Verification items for the finished model (mm, model axes). A direction names the side the tool comes from. Round coordinates to 2 decimals unless told otherwise and drop trailing zeros. Write each loop counter-clockwise with the first axis right and the second up, starting at its lowest first coordinate (ties: lowest second). Pieces come first, ordered by that corner, then holes. Notation, with made-up numbers: M -36,53.5 L -30,53.5 A33 ccw -30,83.5 Z; hole C 72.5,-24 d10. An arc over 180 degrees is marked long. One line per question, with ' | ' between items.
from build123d import *

# Parameters (mm, degrees)
F0_W     = 48.26
F0_H     = 38.1
F1_DEPTH = 15.24
F3_T     = -0.254
F4_D     = 6.858
F6_D     = 5.08
F7_W     = 8.128
F7_H     = 3.048
F8_DEPTH = 25.4


with BuildPart() as f1:
    # F0 (on Front) → F1 (new body)
    with BuildSketch(Plane.XZ):
        Rectangle(F0_W, F0_H)
    extrude(amount=F1_DEPTH)

    # F3
    f3_openings = [f1.faces().sort_by_distance(p)[0] for p in [
        (0, 0, 0),
    ]]
    offset(amount=F3_T, openings=f3_openings)

    # F4 (through all)
    with Locations(Plane.XZ.offset(15.24)):
        with Locations((-16.383, 0)):
            Hole(F4_D / 2)

    # F6 (through all)
    with Locations(Plane.XZ.offset(15.24)):
        with Locations((0, 0)):
            Hole(F6_D / 2)

    # F7 (on face) → F8 (cut)
    with BuildSketch(Plane.XY.offset(19.05)):
        with Locations((16.256, -11.051697)):
            Rectangle(F7_W, F7_H)
    extrude(amount=-F8_DEPTH, mode=Mode.SUBTRACT)


solid = f1.part
1. Section check C-C, the plane y = -3.5. Record the cut outline in (x, z).
Results:
outline: M -24.13,-19.05 L 24.13,-19.05 L 24.13,19.05 L -24.13,19.05 Z; hole M -23.88,-18.8 L 23.88,-18.8 L 23.88,18.8 L -23.88,18.8 Z
2. Section check D-D, the plane x = -9.5. Record the cut outline in (y, z), then the cut area to 3 significant figures.
Results:
outline: M -15.24,-19.05 L 0,-19.05 L 0,-18.8 L -14.99,-18.8 L -14.99,18.8 L 0,18.8 L 0,19.05 L -15.24,19.05 Z | area: 17.3 mm2
3. Section check B-B, the plane x = 0. Record the cut outline in (y, z).
Results:
outline: M -15.24,-19.05 L 0,-19.05 L 0,-18.8 L -14.99,-18.8 L -14.99,-2.54 L -15.24,-2.54 Z; M -15.24,2.54 L -14.99,2.54 L -14.99,18.8 L 0,18.8 L 0,19.05 L -15.24,19.05 Z
4. Section check A-A, the plane z = 0. Record the cut outline in (x, y), then the cut area to 3 significant figures.
Results:
outline: M -24.13,-15.24 L -19.81,-15.24 L -19.81,-14.99 L -23.88,-14.99 L -23.88,0 L -24.13,0 Z; M -12.95,-15.24 L -2.54,-15.24 L -2.54,-14.99 L -12.95,-14.99 Z; M 2.54,-15.24 L 24.13,-15.24 L 24.13,0 L 23.88,0 L 23.88,-14.99 L 2.54,-14.99 Z | area: 16.8 mm2
5. Mould release check, pull along Z, two halves, no side actions. Record for faces 3 (the face through (-24.13, -8, 0)), 4 (the face through (0, -7, 18.796)), 5 (the face through (0, -8, -19.05)), 6 (the face through (-23.876, -7, 0)): pulls with the +Z half, pulls with the -Z half, needs draft (parallel to the pull), parting line crosses it, or undercut.
Results:
face 3: needs draft | face 4: undercut | face 5: pulls with the -Z half | face 6: undercut
6. Go/stop test with a flat-tipped pin: P1, Ø11.5, axis at x = 10, z = 1, coming from the +Y side. Record where the tip stops, or that it passes through.
Results:
P1: stops at y = -14.99
7. Thickness scan on line 1 (X direction, y = -5, z = 15); line 2 (Z direction, x = 0, y = -15.1); line 3 (Z direction, x = 19, y = -7.5). Record the ranges inside material, lowest first.
Results:
line 1: x = -24.13 to -23.88, 23.88 to 24.13 | line 2: z = -19.05 to -2.54, 2.54 to 19.05 | line 3: z = -19.05 to -18.8, 18.8 to 19.05
8. Tool access check on faces 1 (the face through (23.876, -7, 0)), 2 (the face through (0, -8, 19.05)). Record the directions out of +Z, -Z, +X, -X, +Y, -Y that give a thin tool (end or side, any length) a straight path to the whole face; none if there is none.
Results:
face 1: +Y | face 2: +Z, +X, -X, +Y, -Y
